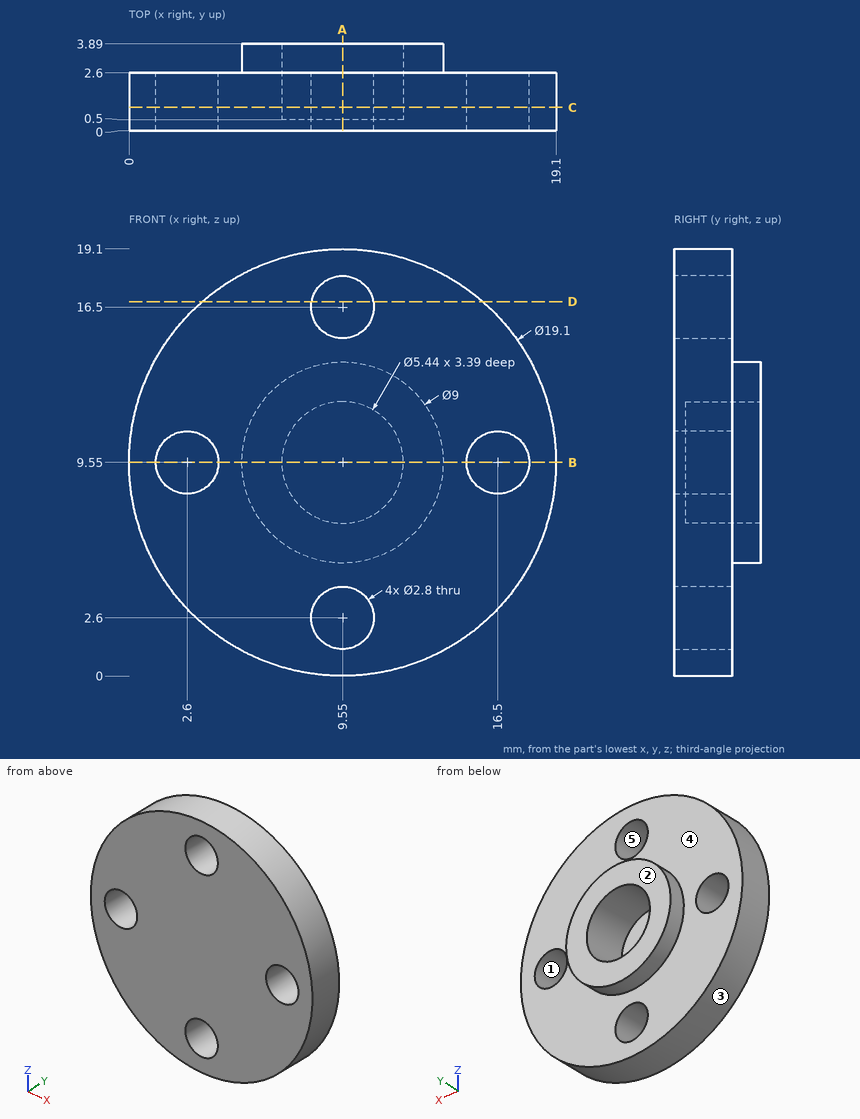
Print and shaded views of the part. All mm, measured from the part's lowest x, y and z. A direction names the side the tool comes from. Coordinates: 2 decimals unless noted, no trailing zeros. Write each loop counter-clockwise with the first axis right and the second up, starting at its lowest first coordinate (ties: lowest second). Pieces come first, ordered by that corner, then holes. Notation, with made-up numbers: M 58.25,-37.5 L 99.25,-37.5 A28 cw 99.25,-9.5 Z; hole C 16,12 d7. An arc over 180 degrees is marked long. Return JSON: item names as keys, results as strings.
1. Flat gauge pins, fed straight in: pin 1 Ø2.5 at (x, z) = (10.5, 10.5) entering from +Y; pin 2 Ø1.5 at (x, y) = (5, 3) entering from -Z; pin 3 Ø6 at (x, z) = (6.5, 2.5) entering from +Y. Where does each tip first touch, or does it go through?
Determined:
{"pin 1": "y = 0.5", "pin 2": "z = 0.84", "pin 3": "y = 2.6"}
2. 3-axis set-ups, long thin cutter, end or side, ignore diameter. For the marked faces 4 and 5: which of +Z, -Z, +X, -X, +Y, -Y reach the whole face in a straight line?
Determined:
{"face 4": "+Y", "face 5": "+Y, -Y"}
3. Pull direction Z, two halves, no side cores. Call the marked faces 1, 2 and 3: pulls with the +Z half, pulls with the -Z half, needs draft (parallel to the pull), parting line crosses it, or undercut.
Determined:
{"face 1": "undercut", "face 2": "needs draft", "face 3": "parting line crosses it"}
4. Saw through at D-D, the plane z = 16.75. Write the cut outline in (x, y), then the cut area to 3 significant figures.
Determined:
{"outline": "M 3.28,0 L 8.17,0 L 8.17,2.6 L 3.28,2.6 Z; M 10.93,0 L 15.82,0 L 15.82,2.6 L 10.93,2.6 Z", "area": "25.5 mm²"}
5. Saw through at B-B, the plane z = 9.55. Write the cut outline in (x, y), then the cut area to 3 significant figures.
Determined:
{"outline": "M 0,0 L 1.2,0 L 1.2,2.6 L 0,2.6 Z; M 4,0 L 15.1,0 L 15.1,2.6 L 14.05,2.6 L 14.05,3.89 L 12.27,3.89 L 12.27,0.5 L 6.83,0.5 L 6.83,3.89 L 5.05,3.89 L 5.05,2.6 L 4,2.6 Z; M 17.9,0 L 19.1,0 L 19.1,2.6 L 17.9,2.6 Z", "area": "28.3 mm²"}
6. Saw through at C-C, the plane y = 1.05. Write the cut outline in (x, z), then the cut area to 3 significant figures.
Determined:
{"outline": "C 9.55,9.55 d19.1; hole C 2.6,9.55 d2.8; hole C 9.55,9.55 d5.44; hole C 9.55,2.6 d2.8; hole C 9.55,16.5 d2.8; hole C 16.5,9.55 d2.8", "area": "239 mm²"}
7. Probe L1, parallel to X at y = 1.95, z = 9.55; L2, parallel to X at y = 0.8, z = 10.5; L3, parallel to Y at x = 6, z = 16.75. List the from-to ranges inside material, lowest first.
Determined:
{"L1": "0 to 1.2, 4 to 6.83, 12.27 to 15.1, 17.9 to 19.1", "L2": "0.05 to 1.57, 3.63 to 7, 12.1 to 15.47, 17.53 to 19.05", "L3": "0 to 2.6"}
8. Saw through at A-A, the plane x = 9.55. Write the cut outline in (y, z).
Determined:
{"outline": "M 0,0 L 2.6,0 L 2.6,1.2 L 0,1.2 Z; M 0,4 L 2.6,4 L 2.6,5.05 L 3.89,5.05 L 3.89,6.83 L 0.5,6.83 L 0.5,12.27 L 3.89,12.27 L 3.89,14.05 L 2.6,14.05 L 2.6,15.1 L 0,15.1 Z; M 0,17.9 L 2.6,17.9 L 2.6,19.1 L 0,19.1 Z"}
